Autodesk Fusion 360 part; units mm, degrees
sketch "Sketch1" plane through (0, -7.0615, 37.6569) normal (0, 0.1843, -0.9829) x (-1, 0, 0)
  line L0 (2.114, 30.6323) -> (-81.886, 30.6323)
  line L1 (-81.886, 30.6323) -> (-81.886, 20.8412)
  line L2 (-81.886, 20.8412) -> (-78.636, 20.8412)
  line L3 (-78.636, 20.8412) -> (-78.636, 28.8412)
  line L4 (-78.636, 28.8412) -> (-6.636, 28.8412)
  line L5 (-6.636, 28.8412) -> (-6.636, -7.4588)
  line L6 (-6.636, -7.4588) -> (-78.636, -7.4588)
  line L7 (-78.636, -7.4588) -> (-78.636, 0.5412)
  line L8 (-78.636, 0.5412) -> (-81.886, 0.5412)
  line L9 (-81.886, 0.5412) -> (-81.886, -10.9695)
  ellipse E0 centre (-79.886, -13.2445) end of major axis (-79.886, -16.2968) minor radius 3 (-76.9458, -12.6383) -> (-81.886, -10.9695) ccw
  line L10 (-76.9458, -12.6383) -> (-76.9458, -9.6383)
  line L11 (-76.9458, -9.6383) -> (-2.8262, -9.6383)
  line L12 (-2.8262, -9.6383) -> (-2.8262, -12.6383)
  ellipse E1 centre (0.114, -13.2445) end of major axis (0.114, -16.2968) minor radius 3 (2.114, -10.9695) -> (-2.8262, -12.6383) ccw
  line L13 (2.114, -10.9695) -> (2.114, 30.6323)
  line L14 (-78.636, 0.5412) -> (-78.636, -7.4588)
  line L15 (-78.636, -7.4588) -> (-6.636, -7.4588)
  line L16 (-6.636, -7.4588) -> (-6.636, 28.8412)
  line L17 (-6.636, 28.8412) -> (-78.636, 28.8412)
  line L18 (-78.636, 28.8412) -> (-78.636, 20.8412)
  line L19 (-78.636, 20.8412) -> (-81.886, 20.8412)
  line L20 (-81.886, 20.8412) -> (-81.886, 0.5412)
  line L21 (-81.886, 0.5412) -> (-78.636, 0.5412)
  line L22 (-70.636, 26.6912) -> (-9.136, 26.6912)
  line L23 (-9.136, 26.6912) -> (-9.136, -5.3088)
  line L24 (-9.136, -5.3088) -> (-70.636, -5.3088)
  line L25 (-70.636, -5.3088) -> (-70.636, 26.6912)
  line L26 (-76.9458, -9.6383) -> (-81.886, -9.6383)
  line L27 (-2.8262, -9.6383) -> (2.114, -9.6383)
  line L28 (-78.636, 20.8412) -> (-78.636, 0.5412)
extrude "Extrude1" add sketch "Sketch1" along normal blind 1.6 contours L0 L1 L2 L3 L4 L5 L6 L7 L8 L9 L11 L13 L14 L15 L16 L17 L18 L19 L21 L26 L27 | L3 L4 L5 L6 L7 L14 L15 L16 L17 L18 L28 | L22 L23 L24 L25
extrude "Extrude2" cut 1 faces at (53.886, 23.2426, 42.2544) along direction (0, -0.982868, -0.18431) blind 0.05
extrude "Extrude3" cut 1 faces at (53.886, -16.4364, 35.3563) along direction (0, 0.982868, 0.18431) blind 0.05
extrude "Extrude4" cut 1 faces at (53.886, 23.1934, 42.2452) along direction (0, -0.982868, -0.18431) blind 0.05
extrude "Extrude5" cut 1 faces at (53.886, -16.3873, 35.3655) along direction (0, 0.982868, 0.18431) blind 0.05
extrude "Extrude6" cut 1 faces at (53.886, -16.3382, 35.3747) along direction (0, 0.982868, 0.18431) blind 0.5
extrude "Extrude7" cut 1 faces at (53.886, 23.1443, 42.236) along direction (0, -0.982868, -0.18431) blind 0.5
extrude "Extrude8" add 1 faces at (53.886, 22.6528, 42.1438) along direction (0, 0.982868, 0.18431) blind 0.2
extrude "Extrude9" add 1 faces at (53.886, -15.8467, 35.4669) along direction (0, -0.982868, -0.18431) blind 0.2
Geometry check sheet. Reference: the model listing, model coordinates, mm. A direction names the side the tool comes from. Give positions to 0.01 mm unless a question says otherwise; leave off trailing zeros. Write each loop counter-clockwise with the first axis right and the second up, starting at its lowest first coordinate (ties: lowest second). Pieces come first, ordered by that corner, then holes.
1) Access from +Z, -Z, +X, -X, +Y, -Y to the whole of each face (thin tool, end or side, straight path). Record for faces 1 (the flat face through (80.238, -6.384, 36.981)), 2 (the flat face through (81.886, 18, 42)), 3 (the flat face through (80.28, 13.57, 40.72)).
2) Section check A-A, the plane x = 24.5. Record the boundary of the cut face in (y, z).
3) Section check C-C, the plane z = 39. Record the boundary of the cut face in (x, y).
4) Material ranges on L1, parallel to X at y = 0.5, z = 38.5; L2, parallel to Z at x = 43, y = 8; L3, parallel to Z at x = 36.5, y = -11, recorded low to high.
5) Section check B-B, the plane y = 9. Record the boundary of the cut face in (x, z), and give its area (3 significant figures).
6) Gauge pin test, flat ends, axial feed: pin 1 (4.5 mm diameter, centred on y = -0.5, z = 38, fed in from +X); pin 2 (6 mm diameter, centred on x = 60.5, y = -7.5, fed in from -Z); pin 3 (1.5 mm diameter, centred on x = 34, y = 10, fed in from +Z). Record the tip position at first contact, or that the pin passes through.
Computed:
1. face 1: +Z, +X, +Y
1. face 2: +Z, -Z, +X, +Y, -Y
1. face 3: -Z, +X, -Y
2. outline: (-16.14, 35.95) - (-15.85, 34.38) - (-15.65, 34.42) - (22.75, 41.62) - (22.95, 41.66) - (22.65, 43.23) - (22.46, 43.19) - (-15.94, 35.99) - close
3. outline: (-2.11, 0.1) - (78.64, 0.1) - (78.64, 8.78) - (-2.11, 8.78) - close
4. L1: x = -2.11 to 78.64
4. L2: z = 38.85 to 40.48
4. L3: z = 35.29 to 36.92
5. outline: (-2.11, 39.04) - (78.64, 39.04) - (78.64, 40.67) - (-2.11, 40.67) - close
5. area: 131 mm2
6. pin 1: stops at x = 78.64
6. pin 2: stops at z = 35.38
6. pin 3: stops at z = 41
